Answer from the drawing. Dimensions are ordinates in mm from the lowest x, y and z of the part. Round coordinates to 2 decimals unless told otherwise and drop trailing zeros. Loops run counter-clockwise (first coordinate to the right, second up) from the corner with the lowest first, then second, coordinate; pieces in that order, holes last. Notation, with made-up numbers: M 48.5,-0.75 L 86.5,-0.75 A22 ccw 86.5,25.25 Z; hole C -31,32 d10. An arc over 180 degrees is marked long. One line per item, written item: value.
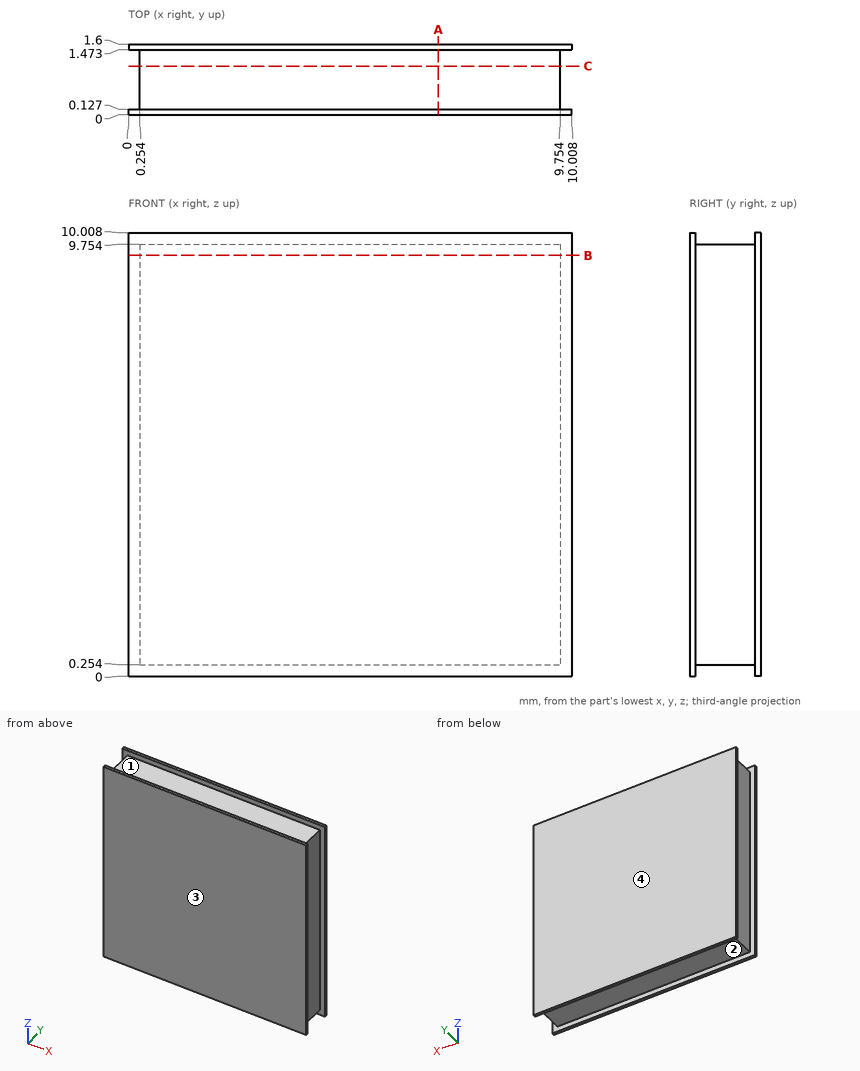
1) Find section C-C (y = 1.1). Give the vertices of the cut face in (x, z).
Check values:
outline: M 0.25,0.25 L 9.75,0.25 L 9.75,9.75 L 0.25,9.75 Z
2) Find section B-B (z = 9.5). Give the vertices of the cut face in (x, y), then the cut area to 3 significant figures.
Check values:
outline: M 0,0 L 10.01,0 L 10.01,0.13 L 9.75,0.13 L 9.75,1.47 L 10.01,1.47 L 10.01,1.6 L 0,1.6 L 0,1.47 L 0.25,1.47 L 0.25,0.13 L 0,0.13 Z
area: 15.3 mm2
3) Find the intervals of material crossed by probe 1 along X at (y, z) = (1.15, 1), in increasing order. Write a range as from..to.
Check values:
probe 1: 0.25..9.75
4) Find section A-A (x = 7). Give the vertices of the cut face in (y, z), then the cut area to 3 significant figures.
Check values:
outline: M 0,0 L 0.13,0 L 0.13,0.25 L 1.47,0.25 L 1.47,0 L 1.6,0 L 1.6,10.01 L 1.47,10.01 L 1.47,9.75 L 0.13,9.75 L 0.13,10.01 L 0,10.01 Z
area: 15.3 mm2
5) Each of these flat-tipped pins is pushed along its axis until it touches: pin 1 (3 mm diameter, centred on x = 7.5, z = 4.5, fed in from -Y); pin 2 (0.7 mm diameter, centred on x = 6, y = 1, fed in from +Z). Where does it stop, or does it pass through?
Check values:
pin 1: y = 0
pin 2: z = 9.75
6) The mould has two halves that part along Y. Classify the marked faces 1, 2, 3 and 4: +Y half, -Y half, draft (parallel to the pull), parting line (faces both ways), or undercut.
Check values:
face 1: undercut
face 2: undercut
face 3: -Y half
face 4: +Y half
